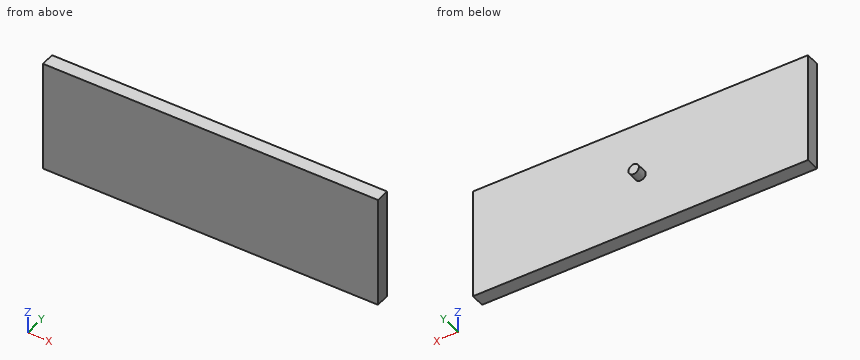
from build123d import *

# Parameters (mm, degrees)
F1_W     = 404.8252
F1_H     = 135.7376
F2_DEPTH = 16.6624
F3_R     = 6.35
F4_DEPTH = 12.7


# Not quite as in the source:
# - a variable given as a bare number and used for a length is read in inches; the dataset says mm whatever the document's units were


with BuildPart() as f2:
    # F1 (on Front) → F2 (new body)
    with BuildSketch(Plane.XZ):
        with Locations((-202.4126, 67.8688)):
            Rectangle(F1_W, F1_H)
    extrude(amount=F2_DEPTH)

    # F3 (on face) → F4 (join)
    with BuildSketch(Plane(origin=(0, 0, 0), x_dir=(-1, 0, 0), z_dir=(0, 1, 0))):
        with Locations((202.4126, 67.8688)):
            Circle(F3_R)
    extrude(amount=F4_DEPTH)


solid = f2.part
Source: CAD feature listing. Evaluate the final solid. Frame: model axes, mm. Round coordinates to 2 decimals unless told otherwise and drop trailing zeros. Write each loop counter-clockwise with the first axis right and the second up, starting at its lowest first coordinate (ties: lowest second). Pieces come first, ordered by that corner, then holes. Notation, with made-up numbers: M 61.5,83.5 L 79.5,83.5 A10 ccw 79.5,93.5 Z; hole C -10,63 d3. An arc over 180 degrees is marked long. One line per item, written item: value. Start each with the question number.
Item 1: Ray query, L1, parallel to Y at x = -322, z = 98. Return the intervals inside material, ascending. Write a range as from..to.
Item 2: Pin query (flat end, axial travel): pin 1 (1 mm diameter, centred on x = -239.5, y = 1.5, fed in from +Z); pin 2 (1 mm diameter, centred on x = -87.5, z = 52.5, fed in from +Y). Return the tip coordinate at first contact, or that it passes through.
Item 3: Section query C-C (y = 7). Return the cut outline in (x, z), plus the area to 3 significant figures.
Item 4: Section query B-B (z = 11). Return the cut outline in (x, y).
Item 5: Section query A-A (x = -173). Return the cut outline in (y, z).
Result set:
1. L1: y = -16.66..0
2. pin 1: passes through
2. pin 2: stops at y = 0
3. outline: C -202.41,67.87 d12.7
3. area: 127 mm²
4. outline: M -404.83,-16.66 L 0,-16.66 L 0,0 L -404.83,0 Z
5. outline: M -16.66,0 L 0,0 L 0,135.74 L -16.66,135.74 Z
